```python
from build123d import *

# Parameters (mm, degrees)
F0_W     = 238.125
F0_H     = 168.275
F1_DEPTH = 6.35
F2_W     = 179.832
F2_H     = 44.958
F3_DEPTH = 25.4
F5_DEPTH = 6.351


# Not quite as in the source:
# - a feature of the source that left no trace in its solid (it failed there, or was rolled back) is left out


with BuildPart() as f1:
    # F0 (on Top) → F1 (new body)
    with BuildSketch(Plane.XY):
        Rectangle(F0_W, F0_H)
    extrude(amount=F1_DEPTH)

    # F2 (on face) → F3 (cut)
    with BuildSketch(Plane.XY.offset(6.35)):
        Rectangle(F2_W, F2_H)
    extrude(amount=-F3_DEPTH, mode=Mode.SUBTRACT)

    # F4 (on face) → F5 (cut, through all)
    with BuildSketch(Plane.XY.offset(6.35)):
        with BuildLine():
            Line((90.3986, 23.749), (-90.3986, 23.749))
            ThreePointArc((-90.3986, 23.749), (-90.9553758795, 23.5183758795), (-91.186, 22.9616))
            Line((-91.186, 22.9616), (-91.186, -22.9616))
            ThreePointArc((-91.186, -22.9616), (-90.9553758795, -23.5183758795), (-90.3986, -23.749))
            Line((-90.3986, -23.749), (90.3986, -23.749))
            ThreePointArc((90.3986, -23.749), (90.9553758795, -23.5183758795), (91.186, -22.9616))
            Line((91.186, -22.9616), (91.186, 22.9616))
            ThreePointArc((91.186, 22.9616), (90.9553758795, 23.5183758795), (90.3986, 23.749))
        make_face()
    extrude(amount=-F5_DEPTH, mode=Mode.SUBTRACT)


solid = f1.part
```
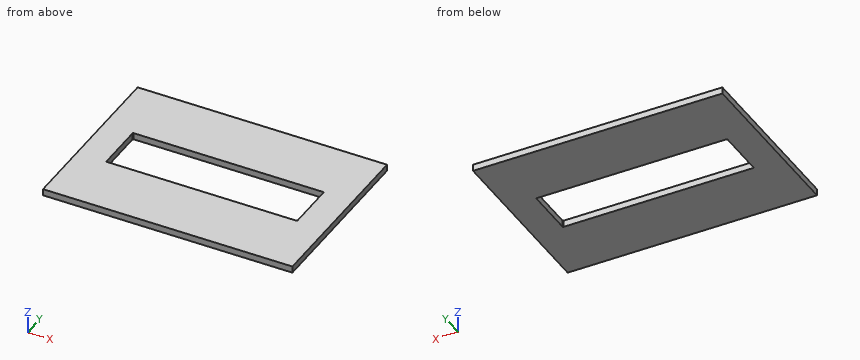
Geometry check sheet. Reference: the model listing, model coordinates, mm. Round coordinates to 2 decimals unless told otherwise and drop trailing zeros. Write each loop counter-clockwise with the first axis right and the second up, starting at its lowest first coordinate (ties: lowest second). Pieces come first, ordered by that corner, then holes. Notation, with made-up numbers: (86, 63) -> (111, 63) arc R18 ccw to (111, 71) -> close; hole circle Ø4 at (54.25, 77.5). An arc over 180 degrees is marked (long way). Put each result on its own line as item: value.
1) Thickness scan on probe 1 along Y at (x, z) = (-34, 2.25); probe 2 along X at (y, z) = (19.5, 6). Record the ranges inside material, lowest first. Write a range as from..to.
Recorded:
probe 1: y = -84.14..-23.75, 23.75..84.14
probe 2: x = -119.06..-91.19, 91.19..119.06
2) Cross-section at B-B, the plane y = 18.5. Enter the section's corners in (x, z), plus the area to 3 significant figures.
Recorded:
outline: (-119.06, 0) -> (-91.19, 0) -> (-91.19, 6.35) -> (-119.06, 6.35) -> close; (91.19, 0) -> (119.06, 0) -> (119.06, 6.35) -> (91.19, 6.35) -> close
area: 354 mm2
3) Cross-section at A-A, the plane x = -85. Enter the section's corners in (y, z).
Recorded:
outline: (-84.14, 0) -> (-23.75, 0) -> (-23.75, 6.35) -> (-84.14, 6.35) -> close; (23.75, 0) -> (84.14, 0) -> (84.14, 6.35) -> (23.75, 6.35) -> close
4) Cross-section at C-C, the plane z = 3. Enter the section's corners in (x, y), plus the area to 3 significant figures.
Recorded:
outline: (-119.06, -84.14) -> (119.06, -84.14) -> (119.06, 84.14) -> (-119.06, 84.14) -> close; hole (-91.19, -22.96) arc R0.79 ccw to (-90.4, -23.75) -> (90.4, -23.75) arc R0.79 ccw to (91.19, -22.96) -> (91.19, 22.96) arc R0.79 ccw to (90.4, 23.75) -> (-90.4, 23.75) arc R0.79 ccw to (-91.19, 22.96) -> close
area: 31,400 mm2
